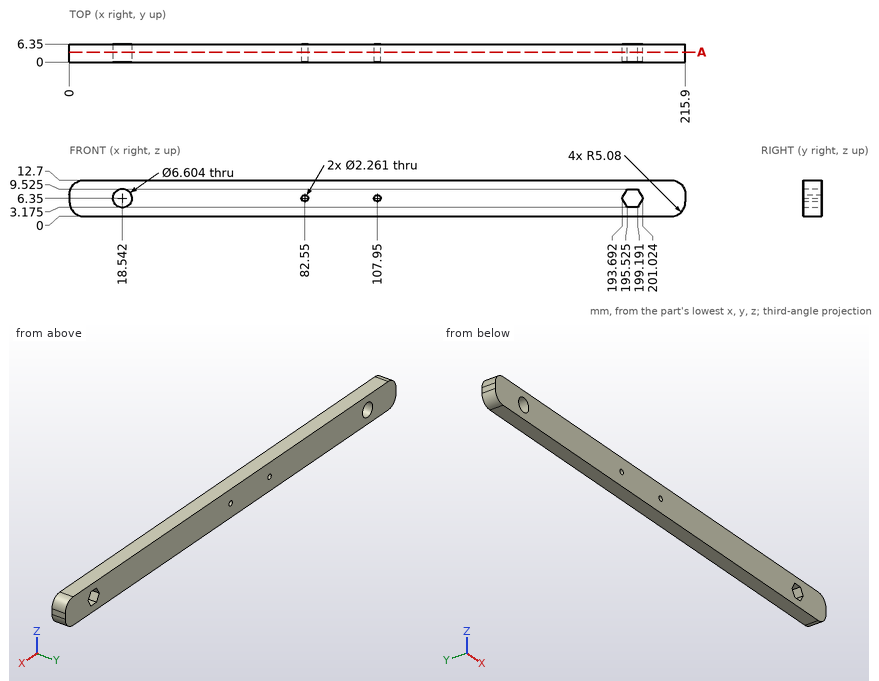
The figure shows three views and two pictorial views of one solid part (mm, origin at its lowest corner). Answer the questions. Round coordinates to 2 decimals unless told otherwise and drop trailing zeros.
Q1. Find the intervals of material crossed by line 1 along X through (y, z) = (3.25, 6.35) (1 decimal); line 2 along X through (y, z) = (1, 7.25) (1 decimal); line 3 along Z through (x, y) = (82.55, 3.75), in increasing order.
Solution:
line 1: x = 0 to 15.2, 21.8 to 81.4, 83.7 to 106.8, 109.1 to 193.7, 201 to 215.9
line 2: x = 0 to 15.4, 21.7 to 81.9, 83.2 to 107.3, 108.6 to 194.2, 200.5 to 215.9
line 3: z = 0 to 5.22, 7.48 to 12.7
Q2. A cutting plane is placed at A-A, the plane y = 3.5. Count the separate pieces of the cut face and the enclosed holes in it, then the cut area to 3 significant figures.
Solution:
separate pieces: 1
enclosed holes: 4
area: 2,640 mm2
Q3. Given pin 1 Ø3 at (y, z) = (4, 2.5) entering from +X, flat-ended and moving along its own axis, determine where the tip first touches the part or whether it passes through.
Solution:
pin 1: stops at x = 215.78
